```python
from build123d import *

# Parameters (mm, degrees)
SKETCH1_W           = 25.4
SKETCH1_H           = 25.4
SKETCH1_R           = 6.35
BOSS_EXTRUDE1_DEPTH = 16.93418
BOSS_EXTRUDE2_DEPTH = 25.4
FILLET1_R           = 6.35
CUT_EXTRUDE1_DEPTH  = 39.338661357


with BuildPart() as part:
    # Sketch1 → Boss-Extrude1 (new, symmetric)
    with BuildSketch(Plane.XY):
        Rectangle(SKETCH1_W, SKETCH1_H)
        Circle(SKETCH1_R, mode=Mode.SUBTRACT)
    extrude(amount=BOSS_EXTRUDE1_DEPTH, both=True)

    # Sketch3 → Boss-Extrude2 (add)
    with BuildSketch(Plane(origin=(12.7, 0, 0), x_dir=(0, 0, -1), z_dir=(1, 0, 0))):
        Polygon((-16.93418, -12.7), (-16.93418, 12.7), (-16.93418, 19.05), (-21.489310241, 19.05), (-21.489310241, -19.05), (-16.93418, -19.05), align=None)
        Polygon((16.93418, -12.7), (16.93418, 12.7), (16.93418, 19.05), (21.489310241, 19.05), (21.489310241, -19.05), (16.93418, -19.05), align=None)
    extrude(amount=-BOSS_EXTRUDE2_DEPTH)

    # Fillet1
    fillet1_edges = [part.edges().sort_by_distance(p)[0] for p in [
        (0, -12.7, -16.93418),
        (0, -12.7, 16.93418),
        (0, 12.7, 16.93418),
        (0, 12.7, -16.93418),
    ]]
    fillet(fillet1_edges, radius=FILLET1_R - 0.0001)  # a hair under: the kernel refuses the full size

    # Sketch3<2> → Cut-Extrude1 (cut, through all)
    with BuildSketch(Plane(origin=(12.7, 0, 0), x_dir=(0, 0, -1), z_dir=(1, 0, 0))):
        Polygon((-16.93418, -12.7), (-16.93418, 12.7), (-16.93418, 19.05), (-21.489310241, 19.05), (-21.489310241, -19.05), (-16.93418, -19.05), align=None)
        Polygon((16.93418, -12.7), (16.93418, 12.7), (16.93418, 19.05), (21.489310241, 19.05), (21.489310241, -19.05), (16.93418, -19.05), align=None)
    extrude(amount=-CUT_EXTRUDE1_DEPTH, mode=Mode.SUBTRACT)


solid = part.part
```
Input: part model. Units: mm. Frame: model coordinates. A direction names the side the tool comes from. Coordinates: 2 decimals unless noted, no trailing zeros. Write each loop counter-clockwise with the first axis right and the second up, starting at its lowest first coordinate (ties: lowest second). Pieces come first, ordered by that corner, then holes. Notation, with made-up numbers: (58.25, 76.25) - (84.25, 76.25) arc R23 cw to (84.25, 88.25) - close; hole circle Ø6 at (29, -2.5). An arc over 180 degrees is marked (long way). Put each result on its own line as item: value. Start each with the question number.
1) Mould query, pull axis Y, two halves, no side actions, for faces 4 (the face through (-1.38, -6.2, -0.24)), 5 (the face through (0.178, 14.609, 15.123)), 6 (the face through (0.178, -14.511, -15.025)). Classes: pulls with the +Y half, pulls with the -Y half, needs draft (parallel to the pull), parting line crosses it, or undercut.
2) Cut plane C-C (z = 3). Return the cut outline in (x, y), plus the area to 3 significant figures.
3) Contact query for flat-ended pins moving along their axis: pin 1 (3 mm diameter, centred on x = 9.5, z = -13, fed in from -Y); pin 2 (10 mm diameter, centred on x = 0, y = 0, fed in from +Z); pin 3 (6.5 mm diameter, centred on x = 5, z = 2, fed in from -Y); pin 4 (6 mm diameter, centred on x = 4, z = 9, fed in from +Y). Output: stop coordinate, or through.
4) Cut plane D-D (y = 14.5). Return the cut outline in (x, z).
5) Cut plane A-A (y = 0). Return the cut outline in (x, z), plus the area to 3 significant figures.
6) Ray query, L1, parallel to Y at x = 0, z = 1; L2, parallel to Y at x = 7.5, z = -3; L3, parallel to Z at x = -7.75, y = -17. Return the intervals inside material, ascending.
7) Reachability of faces 1 (the face through (-5.5, -4, -16.934)), 2 (the face through (0.178, 14.511, -15.025)), 3 (the face through (0, -12.7, 0)) from +Z, -Z, +X, -X, +Y, -Y: full face, straight path, thin tool, end or side. Return the list, or none.
8) Cut plane B-B (x = 0). Return the cut outline in (y, z).
Resolved:
1. face 4: undercut
1. face 5: pulls with the +Y half
1. face 6: pulls with the -Y half
2. outline: (-12.7, -12.7) - (12.7, -12.7) - (12.7, 12.7) - (-12.7, 12.7) - close; hole circle Ø12.7 at (0, 0)
2. area: 518 mm2
3. pin 1: stops at y = -14.05
3. pin 2: passes through
3. pin 3: stops at y = -12.7
3. pin 4: stops at y = 12.86
4. outline: (-12.7, -16.93) - (12.7, -16.93) - (12.7, -15.01) - (-12.7, -15.01) - close; (-12.7, 15.01) - (12.7, 15.01) - (12.7, 16.93) - (-12.7, 16.93) - close
5. outline: (-12.7, -16.93) - (-6.35, -16.93) - (-6.35, 16.93) - (-12.7, 16.93) - close; (6.35, -16.93) - (12.7, -16.93) - (12.7, 16.93) - (6.35, 16.93) - close
5. area: 430 mm2
6. L1: y = -12.7 to -6.35, 6.35 to 12.7
6. L2: y = -12.7 to 12.7
6. L3: z = -16.93 to -16.59, 16.59 to 16.93
7. face 1: -Z, +X, -X, +Y, -Y
7. face 2: +X, -X, +Y
7. face 3: +X, -X, -Y
8. outline: (-19.05, -16.93) - (-6.35, -16.93) - (-6.35, 16.93) - (-19.05, 16.93) arc R6.35 cw to (-12.7, 10.58) - (-12.7, -10.58) arc R6.35 cw to start; (6.35, -16.93) - (19.05, -16.93) arc R6.35 cw to (12.7, -10.58) - (12.7, 10.58) arc R6.35 cw to (19.05, 16.93) - (6.35, 16.93) - close
